The listing builds one solid part. Answer for the finished solid, in the listing's coordinates (mm). A direction names the side the tool comes from. Round coordinates to 2 decimals unless told otherwise and drop trailing zeros. Answer as a JSON object with one key per item and string values.
```python
from build123d import *

# Parameters (mm, degrees)
F1_DEPTH = 9.525
F2_T     = -1.5875
F3_R     = 3.96875
F4_DEPTH = 6.35
F5_R     = 0.79375
F6_R     = 2.38125


with BuildPart() as f1:
    # F0 (on Front) → F1 (new body)
    with BuildSketch(Plane.XZ):
        with BuildLine():
            Line((44.45, 0), (-19.05, 0))
            ThreePointArc((-19.05, 0), (-23.5401280605, -1.8598719395), (-25.4, -6.35))
            Line((-25.4, -6.35), (-25.4, -76.2))
            ThreePointArc((-25.4, -76.2), (-23.5401280605, -80.6901280605), (-19.05, -82.55))
            Line((-19.05, -82.55), (19.05, -82.55))
            Line((19.05, -82.55), (34.1089205608, -73.8557281605))
            ThreePointArc((34.1089205608, -73.8557281605), (36.6961873461, -71.0245713224), (37.1814148685, -67.2201064833))
            ThreePointArc((37.1814148685, -67.2201064833), (37.6995950161, -37.3548976318), (49.6577958893, -9.9833678558))
            ThreePointArc((49.6577958893, -9.9833678558), (50.0800260161, -3.4131126923), (44.45, 0))
        make_face()
    extrude(amount=F1_DEPTH)

    # F2
    f2_openings = [f1.faces().sort_by_distance(p)[0] for p in [
        (7.276457, -9.525, -39.048077),
    ]]
    offset(amount=F2_T, openings=f2_openings)

    # F3 (on face) → F4 (join)
    with BuildSketch(Plane.XZ.offset(1.5875)):
        with Locations((41.275, -9.525)):
            Circle(F3_R)
        with Locations((12.7, -9.525)):
            Circle(F3_R)
        with Locations((30.1625, -34.925)):
            Circle(F3_R)
        with Locations((22.225, -65.0875)):
            Circle(F3_R)
    extrude(amount=F4_DEPTH)

    # F5
    f5_edges = [f1.edges().sort_by_distance(p)[0] for p in [
        (-23.8125, -1.5875, -41.275),
    ]]
    fillet(f5_edges, radius=F5_R)

    # F6
    f6_edges = [f1.edges().sort_by_distance(p)[0] for p in [
        (37.699595, 0, -37.354898),
    ]]
    fillet(f6_edges, radius=F6_R)


solid = f1.part
```
Item 1: Straight lines are drawn through the part: line 1 (Z direction, x = 4, y = -4); line 2 (X direction, y = -3.5, z = -37.5); line 3 (Z direction, x = -19.5, y = -3.5). For each, find the intervals that lie inside material, in ascending order.
Values follow:
{"line 1": "-82.55 to -80.96, -1.59 to 0", "line 2": "-25.4 to -23.81, 27.14 to 33.18, 36.04 to 37.67", "line 3": "-82.53 to -80.94, -1.61 to -0.02"}
Item 2: Determine the mould class of faces 3 (the face through (4, -1.588, -41)), 4 (the face through (26.474, -5.903, -78.264)), 5 (the face through (4, 0, -41)) for opening direction X: released by +X, released by -X, zero draft, split by the parting line, or undercut.
Values follow:
{"face 3": "undercut", "face 4": "released by +X", "face 5": "zero draft"}
Item 3: The part is cut by section B-B (y = -4.25). Give the number of separate pieces and of enclosed holes in the cut face, then the cut area to 3 significant figures.
Values follow:
{"separate pieces": "5", "enclosed holes": "1", "area": "651 mm^2"}
Item 4: Which of the six approach directions +Z, -Z, +X, -X, +Y, -Y give full straight-line access (tool end or side, diameter ignored) to faces 1 (the face through (-25.4, -6, -41)), 2 (the face through (0, -6, -80.962))?
Values follow:
{"face 1": "+Z, -Z, -X, +Y, -Y", "face 2": "-Y"}
Item 5: Flat-ended cylindrical pins translate along their axes: P1, Ø5, axis at x = 12, z = -12.5, coming from the -Y side; P2, Ø4, axis at y = -6.5, z = -59, coming from the +X side; P3, Ø5, axis at y = -4, z = -67.5, coming from the +X side. Find the tip coordinate at first contact, or state that the pin passes through.
Values follow:
{"P1": "y = -7.94", "P2": "x = 36.31", "P3": "x = 37.28"}
